from build123d import *

# Parameters (mm, degrees)
SKETCH2_W           = 101.6
SKETCH2_H           = 17.78
BOSS_EXTRUDE1_DEPTH = 3.175
BOSS_EXTRUDE2_DEPTH = 7.62
BOSS_EXTRUDE3_DEPTH = 38.1
FILLET2_R           = 2.54
FILLET3_R           = 2.54
SKETCH6_R           = 1.4605
CUT_EXTRUDE1_DEPTH  = 161.318129994


with BuildPart() as part:
    # Sketch2 → Boss-Extrude1 (new body)
    with BuildSketch(Plane(origin=(0, 0, 0), x_dir=(1, 0, 0), z_dir=(0, 1, 0))):
        with Locations((50.8, 8.89)):
            Rectangle(SKETCH2_W, SKETCH2_H)
    boss_extrude1 = extrude(amount=BOSS_EXTRUDE1_DEPTH)

    # Sketch3 → Boss-Extrude2 (add)
    with BuildSketch(Plane.XZ):
        with BuildLine():
            Line((93.98, -14.351), (5.08, -14.351))
            ThreePointArc((5.08, -14.351), (1.905, -11.176), (5.08, -8.001))
            Line((5.08, -8.001), (93.98, -8.001))
            ThreePointArc((93.98, -8.001), (97.155, -11.176), (93.98, -14.351))
        make_face()
    extrude(amount=BOSS_EXTRUDE2_DEPTH)

    # Mirror1: Boss-Extrude1 across plane
    add(boss_extrude1.mirror(Plane(origin=(0, -3.81, 0), x_dir=(0, 0, 1), z_dir=(0, -1, 0))))

    # Sketch5 → Boss-Extrude3 (add)
    with BuildSketch(Plane.XZ.offset(10.795)):
        with BuildLine():
            Line((0, 0), (13.724447784, 0))
            Line((13.724447784, 0), (13.724447784, -118.618))
            ThreePointArc((13.724447784, -118.618), (3.519309988, -98.867872234), (0, -76.917317766))
            Line((0, -76.917317766), (0, 0))
        make_face()
    extrude(amount=BOSS_EXTRUDE3_DEPTH)

    # Fillet2
    fillet2_edges = [part.edges().sort_by_distance(p)[0] for p in [
        (13.724447784, -29.845, -118.618),
    ]]
    fillet(fillet2_edges, radius=FILLET2_R)

    # Fillet3
    # the kernel refuses this fillet: 2.54 mm, written as the material it adds along each edge
    with BuildSketch(Plane(origin=(13.724447784, -10.795, 0), x_dir=(0, -1, 0), z_dir=(0, 0, -1))) as fillet3_piece_1:
        with BuildLine():
            CenterArc((FILLET3_R, -FILLET3_R), FILLET3_R, 90, 90)
            Line((0, -FILLET3_R), (0, 0))
            Line((0, 0), (FILLET3_R, 0))
        make_face()
    extrude(amount=17.78)
    # the kernel refuses this fillet: 2.54 mm, written as the material it takes off along each edge
    with BuildSketch(Plane(origin=(0, -1.27, 0), x_dir=(0, 0, -1), z_dir=(0, -1, 0))) as fillet3_2_piece_1:
        with BuildLine():
            CenterArc((FILLET3_R, FILLET3_R), FILLET3_R, 180, 90)
            Line((0, FILLET3_R), (0, 0))
            Line((0, 0), (FILLET3_R, 0))
        make_face()
    extrude(amount=53.975, mode=Mode.SUBTRACT)
    with BuildSketch(Plane(origin=(-6.35, -48.895, 0), x_dir=(0, 0, -1), z_dir=(1, 0, 0))) as fillet3_2_piece_2:
        with BuildLine():
            CenterArc((FILLET3_R, FILLET3_R), FILLET3_R, 180, 90)
            Line((0, FILLET3_R), (0, 0))
            Line((0, 0), (FILLET3_R, 0))
        make_face()
    extrude(amount=26.424447784, mode=Mode.SUBTRACT)

    # Sketch6 → Cut-Extrude1 (cut, through all)
    with BuildSketch(Plane(origin=(0, 3.175, 0), x_dir=(1, 0, 0), z_dir=(0, 1, 0))):
        with Locations(Location((88.9, 11.049, 0), (0, 0, 270))):
            Circle(SKETCH6_R)
        with Locations(Location((33.02, 11.049, 0), (0, 0, 270))):
            Circle(SKETCH6_R)
    extrude(amount=-CUT_EXTRUDE1_DEPTH, mode=Mode.SUBTRACT)


solid = part.part
Geometry: final body of the model. Coordinates: model frame, mm. A direction names the side the tool comes from. Round coordinates to 2 decimals unless told otherwise and drop trailing zeros. Loops run counter-clockwise (first coordinate to the right, second up) from the corner with the lowest first, then second, coordinate; pieces in that order, holes last.
Q1. Section C-C on z = -87. Return loops of the section in (x, y) (3 decimals).
Q2. Section B-B on z = -26. Return loops of the section in (x, y) (3 decimals), plus the area to 3 significant figures.
Q3. Section A-A on x = 33.02. Return loops of the section in (y, z) (1 decimal), plus the area to 3 significant figures.
Q4. Material intervals for L1, parallel to Z at x = 88.9, y = -4.75; L2, parallel to Z at x = 88.9, y = 0.25; L3, parallel to X at y = -13, z = -58, sorted ascending.
Q5. Pin query (flat end, axial travel): P1, Ø9, axis at x = 60, z = -10.5, coming from the -Y side (3 decimals); P2, Ø11, axis at x = 3.5, z = -60.5, coming from the +Y side (3 decimals); P3, Ø2.5, axis at x = 57, y = -3.5, coming from the -Z side. Return the tip coordinate at first contact, or that it passes through.
Q6. Pull-direction query (Y, two-part tool) for faces 6 (the cylindrical face through (97.154, -3.757, -11.106)), 7 (the flat face through (13.724, -30, -54)), 8 (the flat face through (58, -10.795, -9)); classes: released by +Y, released by -Y, zero draft, split by the parting line, or undercut.
Q7. Access query for faces 1 (the cylindrical face through (0.764, -27.969, -0.724)), 2 (the flat face through (49, -4, -8.001)), 3 (the flat face through (101.6, 2, -9)), 4 (the cylindrical face through (1.906, -3.757, -11.246)), 5 (the flat face through (7, -48.895, -57)). Directions: +Z, -Z, +X, -X, +Y, -Y. A direction counts if a zero-diameter tool reaches every point of the face in a straight line with its end or side. Return the directions, or none.
Evaluation:
1. outline: (0.728, -48.895) - (13.724, -48.895) - (13.724, -10.795) - (0.728, -10.795) - close
2. outline: (0, -48.895) - (13.724, -48.895) - (13.724, -10.795) - (0, -10.795) - close
2. area: 523 mm2
3. outline: (-10.8, -17.8) - (-7.6, -17.8) - (-7.6, -14.4) - (0, -14.4) - (0, -17.8) - (3.2, -17.8) - (3.2, -12.5) - (-10.8, -12.5) - close; (-10.8, -9.6) - (3.2, -9.6) - (3.2, 0) - (0, 0) - (0, -8) - (-7.6, -8) - (-7.6, 0) - (-10.8, 0) - close
3. area: 120 mm2
4. L1: z = -14.35 to -12.51, -9.59 to -8
4. L2: z = -17.78 to -12.51, -9.59 to 0
4. L3: x = 0 to 13.72
5. P1: stops at y = -10.795
5. P2: stops at y = -10.795
5. P3: stops at z = -14.35
6. face 6: undercut
6. face 7: zero draft
6. face 8: released by -Y
7. face 1: +Z, -X, -Y
7. face 2: +Z, +X, -X
7. face 3: +Z, -Z, +X, +Y, -Y
7. face 4: -X
7. face 5: +Z, -Z, +X, -X, -Y
